Can you work these out from the drawing? Everything is in mm from the part's minimum corner. Round coordinates to 2 decimals unless told otherwise and drop trailing zeros. Loops run counter-clockwise (first coordinate to the right, second up) from the corner with the lowest first, then second, coordinate; pieces in that order, holes last. Notation, with made-up numbers: M -1.5,5 L 45.5,5 A21 cw 45.5,30 Z; hole C -8.5,-28 d7. An arc over 180 degrees is marked long. Answer in a Markdown table with one row per item.
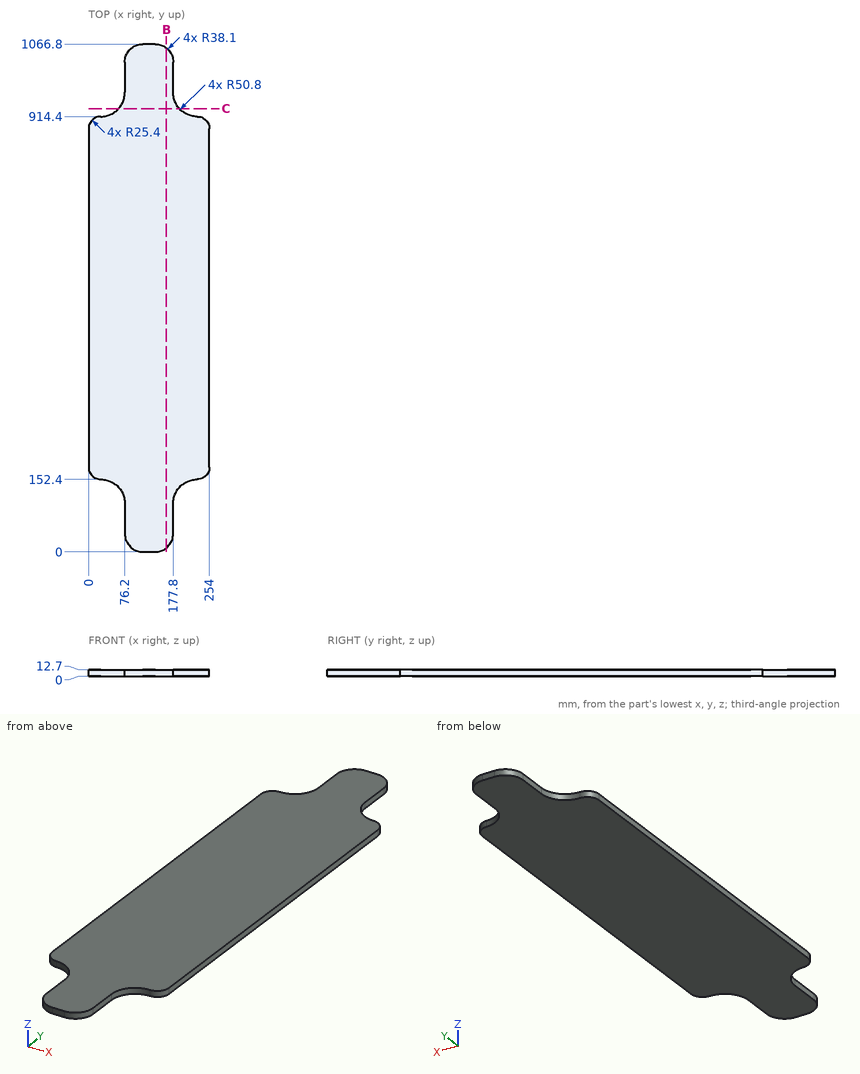
1) I need wall thicknesses on line 1 (X direction, y = 999, z = 10); line 2 (Y direction, x = 222.5, z = 2.75); line 3 (Y direction, x = 20.5, z = 5.5). Which ranges of each line are inside material? Lowest first, please.
Computed:
| item | result |
|---|---|
| line 1 | x = 76.2 to 177.8 |
| line 2 | y = 152.03 to 914.77 |
| line 3 | y = 152.88 to 913.92 |
2) I want a section at C-C, the plane y = 931. Please give me the cut outline in (x, z).
Computed:
| item | result |
|---|---|
| outline | M 62.96,0 L 191.04,0 L 191.04,12.7 L 62.96,12.7 Z |
3) I want a section at B-B, the plane x = 163.5. Please give me the cut outline in (y, z), plus the area to 3 significant figures.
Computed:
| item | result |
|---|---|
| outline | M 8.35,0 L 1058.45,0 L 1058.45,12.7 L 8.35,12.7 Z |
| area | 13,300 mm² |
4) Will these pins go through, and if not, where does the flat tip stop? P1, Ø2, axis at y = 628, z = 2.5, coming from the -X side; P2, Ø4, axis at x = 60.5, z = 10.5, coming from the +Y side; P3, Ø6.5, axis at y = 1003.5, z = 4, coming from the -X side; P4, Ø6.5, axis at y = 60, z = 8, coming from the +X side.
Computed:
| item | result |
|---|---|
| P1 | stops at x = 0 |
| P2 | stops at y = 930.5 |
| P3 | stops at x = 76.2 |
| P4 | stops at x = 177.8 |
